Build history of the part. All positions in model axes, mm. Face numbers are marked on the shaded views. Coordinates: 2 decimals unless noted, no trailing zeros. Loops run counter-clockwise (first coordinate to the right, second up) from the corner with the lowest first, then second, coordinate; pieces in that order, holes last.
Item 1: Drill centre lines: line 1 along Z through (x, y) = (124, 0); line 2 along X through (y, z) = (-25, -33.5); line 3 along Y through (x, z) = (17, 2.5). Where is each one in solid material? Low to high.
Item 2: Cut at A-A (z = 0). List the corners of the cut face in (x, y).
Item 3: Mould opens along Y. For the marked faces 1 and 2 say: released by +Y, released by -Y, zero draft, split by the parting line, or undercut.
Item 4: Flat gauge pins, fed straight in: pin 1 (1.9 mm diameter, centred on x = 166, z = -31.5, fed in from -Y); pin 2 (4.5 mm diameter, centred on x = 166.5, z = 30, fed in from +Y); pin 3 (12.5 mm diameter, centred on y = 21.5, z = 40, fed in from -X); pin 4 (4 mm diameter, centred on x = 138, y = 14.5, fed in from +Z). Where does each tip first touch, or does it go through?
Item 5: Cut at D-D (z = 36). List the corners of the cut face in (x, y).
Item 6: Cut at B-B (y = 21). List the corners of the cut face in (x, z), and give its area (3 significant figures).
Item 7: Cut at C-C (x = -41.5). List the corners of the cut face in (y, z), and give its area (4 significant figures).
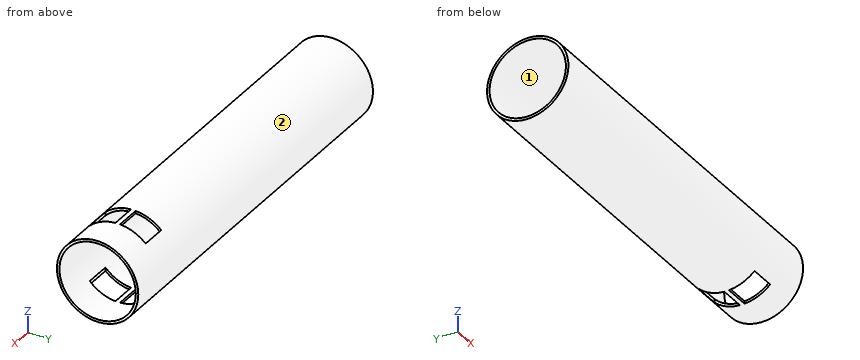
from build123d import *

# Parameters (mm, degrees)
SKETCH12_R              = 44.45
SKETCH12_R_2            = 41.7068
PIPE_0_5_SCH_40_1_DEPTH = 420
CUT_EXTRUDE1_DEPTH      = 50
CUT_EXTRUDE1_DEPTH_BACK = 50
SKETCH13_W              = 28
SKETCH13_H              = 28


with BuildPart() as part:
    # Sketch12 → Pipe 0.5 SCH 40(1) (new body)
    with BuildSketch(Plane.YZ.offset(-210)):
        Circle(SKETCH12_R)
        Circle(SKETCH12_R_2, mode=Mode.SUBTRACT)
    extrude(amount=PIPE_0_5_SCH_40_1_DEPTH)

    # Sketch13 → Cut-Extrude1 (cut, two sides: drawn at the far end of the back side and taken through both)
    with BuildSketch(Plane.XY.offset(-CUT_EXTRUDE1_DEPTH_BACK)):
        with Locations((160, 16.5)):
            Rectangle(SKETCH13_W, SKETCH13_H)
        with Locations((160, -16.5)):
            Rectangle(SKETCH13_W, SKETCH13_H)
    extrude(amount=CUT_EXTRUDE1_DEPTH + CUT_EXTRUDE1_DEPTH_BACK, mode=Mode.SUBTRACT)


solid = part.part
Filled sheet:
1. line 1: z = -44.45 to -41.71, 41.71 to 44.45
1. line 2: x = -210 to 146, 174 to 210
1. line 3: y = -44.38 to -41.63, 41.63 to 44.38
2. outline: (-210, -44.45) - (210, -44.45) - (210, -41.71) - (-210, -41.71) - close; (-210, 41.71) - (210, 41.71) - (210, 44.45) - (-210, 44.45) - close
3. face 1: undercut
3. face 2: split by the parting line
4. pin 1: stops at y = -32.29
4. pin 2: stops at y = 34.72
4. pin 3: stops at x = -210
4. pin 4: stops at z = 42.66
5. outline: (-210, -26.07) - (146, -26.07) - (146, -21.06) - (-210, -21.06) - close; (-210, 21.06) - (146, 21.06) - (146, 26.07) - (-210, 26.07) - close; (174, -26.07) - (210, -26.07) - (210, -21.06) - (174, -21.06) - close; (174, 21.06) - (210, 21.06) - (210, 26.07) - (174, 26.07) - close
6. outline: (-210, -39.18) - (146, -39.18) - (146, -36.03) - (-210, -36.03) - close; (-210, 36.03) - (146, 36.03) - (146, 39.18) - (-210, 39.18) - close; (174, -39.18) - (210, -39.18) - (210, -36.03) - (174, -36.03) - close; (174, 36.03) - (210, 36.03) - (210, 39.18) - (174, 39.18) - close
6. area: 2,460 mm2
7. outline: circle Ø88.9 at (0, 0); hole circle Ø83.41 at (0, 0)
7. area: 742.5 mm2
